For this review, take the finished solid that the model builds, in its own axes (mm). A direction names the side the tool comes from. Round coordinates to 2 decimals unless told otherwise and drop trailing zeros. Order: outer loops, then holes, each group sorted by start corner. A loop starts at its lowest first (then second) coordinate and runs counter-clockwise, first axis right, second up. Notation, with made-up numbers: (67.5, -36.5) -> (106.5, -36.5) arc R26 ccw to (106.5, 2.5) -> close; hole circle Ø10 at (35, 77.25). An arc over 180 degrees is marked (long way). Answer in a Markdown table with one row per item.
```python
from build123d import *

# Parameters (mm, degrees)
F1_DEPTH  = 93
F3_DEPTH  = 25
F4_W      = 122
F4_H      = 3
F4_W_2    = 15
F5_DEPTH  = 15
F6_DEPTH  = 15
F7_DEPTH  = 15
F8_DEPTH  = 15
F9_DEPTH  = 15
F10_DEPTH = 15
F11_DEPTH = 15
F12_DEPTH = 15
F13_DEPTH = 15
F14_DEPTH = 15
F15_DEPTH = 15
F16_DEPTH = 15
F17_DEPTH = 15
F18_DEPTH = 15
F19_W     = 10
F19_H     = 20
F20_DEPTH = 0.2
F21_R     = 2.5
F22_DEPTH = 2
F23_DEPTH = 2
F24_W     = 13
F24_H     = 5
F25_DEPTH = 2


with BuildPart() as f1:
    # F0 (on Top) → F1 (new body)
    with BuildSketch(Plane.XY):
        with BuildLine():
            Line((67.644592, 203.804426), (-232.355408, 203.804426))
            ThreePointArc((-232.355408, 203.804426), (-242.96201, 199.411027), (-247.355408, 188.804426))
            Line((-247.355408, 188.804426), (-247.355408, -176.195574))
            Line((-247.355408, -176.195574), (82.644592, -176.195574))
            Line((82.644592, -176.195574), (82.644592, 188.804426))
            ThreePointArc((82.644592, 188.804426), (78.251193, 199.411027), (67.644592, 203.804426))
        make_face()
        with BuildLine():
            ThreePointArc((-240.355408, 188.804426), (-238.012263, 194.46128), (-232.355408, 196.804426))
            Line((-232.355408, 196.804426), (67.644592, 196.804426))
            ThreePointArc((67.644592, 196.804426), (73.301446, 194.46128), (75.644592, 188.804426))
            Line((75.644592, 188.804426), (75.644592, -169.195574))
            Line((75.644592, -169.195574), (-240.355408, -169.195574))
            Line((-240.355408, -169.195574), (-240.355408, 188.804426))
        make_face(mode=Mode.SUBTRACT)
    extrude(amount=F1_DEPTH)

    # F2 (on face) → F3 (cut)
    with BuildSketch(Plane.XZ.offset(176.195574)):
        Polygon((-30.355408, 6), (72.644592, 6), (72.644592, 100.520082), (-30.355408, 100.520082), (-30.355408, 48), align=None)
        Polygon((-90.355408, 48), (-30.355408, 48), (-30.355408, 100.520082), (-90.355408, 99.808939), align=None)
    extrude(amount=-F3_DEPTH, mode=Mode.SUBTRACT)

    # F4 (on face) → F5 (cut)
    with BuildSketch(Plane(origin=(0, 203.804426, 0), x_dir=(-1, 0, 0), z_dir=(0, 1, 0))):
        with Locations((171.355408, 88.5)):
            Rectangle(F4_W, F4_H)
        with Locations((239.855408, 88.5)):
            Rectangle(F4_W_2, F4_H)
    extrude(amount=-F5_DEPTH, mode=Mode.SUBTRACT)

    # F4 (on face) → F6 (cut)
    with BuildSketch(Plane(origin=(0, 203.804426, 0), x_dir=(-1, 0, 0), z_dir=(0, 1, 0))):
        with Locations((171.355408, 82.5)):
            Rectangle(F4_W, F4_H)
        with Locations((239.855408, 82.5)):
            Rectangle(F4_W_2, F4_H)
    extrude(amount=-F6_DEPTH, mode=Mode.SUBTRACT)

    # F4 (on face) → F7 (cut)
    with BuildSketch(Plane(origin=(0, 203.804426, 0), x_dir=(-1, 0, 0), z_dir=(0, 1, 0))):
        with Locations((171.355408, 76.5)):
            Rectangle(F4_W, F4_H)
        with Locations((239.855408, 76.5)):
            Rectangle(F4_W_2, F4_H)
    extrude(amount=-F7_DEPTH, mode=Mode.SUBTRACT)

    # F4 (on face) → F8 (cut)
    with BuildSketch(Plane(origin=(0, 203.804426, 0), x_dir=(-1, 0, 0), z_dir=(0, 1, 0))):
        with Locations((171.355408, 70.5)):
            Rectangle(F4_W, F4_H)
        with Locations((239.855408, 70.5)):
            Rectangle(F4_W_2, F4_H)
    extrude(amount=-F8_DEPTH, mode=Mode.SUBTRACT)

    # F4 (on face) → F9 (cut)
    with BuildSketch(Plane(origin=(0, 203.804426, 0), x_dir=(-1, 0, 0), z_dir=(0, 1, 0))):
        with Locations((171.355408, 64.5)):
            Rectangle(F4_W, F4_H)
        with Locations((239.855408, 64.5)):
            Rectangle(F4_W_2, F4_H)
    extrude(amount=-F9_DEPTH, mode=Mode.SUBTRACT)

    # F4 (on face) → F10 (cut)
    with BuildSketch(Plane(origin=(0, 203.804426, 0), x_dir=(-1, 0, 0), z_dir=(0, 1, 0))):
        with Locations((171.355408, 58.5)):
            Rectangle(F4_W, F4_H)
        with Locations((239.855408, 58.5)):
            Rectangle(F4_W_2, F4_H)
    extrude(amount=-F10_DEPTH, mode=Mode.SUBTRACT)

    # F4 (on face) → F11 (cut)
    with BuildSketch(Plane(origin=(0, 203.804426, 0), x_dir=(-1, 0, 0), z_dir=(0, 1, 0))):
        with Locations((171.355408, 52.5)):
            Rectangle(F4_W, F4_H)
        with Locations((239.855408, 52.5)):
            Rectangle(F4_W_2, F4_H)
    extrude(amount=-F11_DEPTH, mode=Mode.SUBTRACT)

    # F4 (on face) → F12 (cut)
    with BuildSketch(Plane(origin=(0, 203.804426, 0), x_dir=(-1, 0, 0), z_dir=(0, 1, 0))):
        with Locations((171.355408, 46.5)):
            Rectangle(F4_W, F4_H)
        with Locations((239.855408, 46.5)):
            Rectangle(F4_W_2, F4_H)
    extrude(amount=-F12_DEPTH, mode=Mode.SUBTRACT)

    # F4 (on face) → F13 (cut)
    with BuildSketch(Plane(origin=(0, 203.804426, 0), x_dir=(-1, 0, 0), z_dir=(0, 1, 0))):
        with Locations((171.355408, 40.5)):
            Rectangle(F4_W, F4_H)
        with Locations((239.855408, 40.5)):
            Rectangle(F4_W_2, F4_H)
    extrude(amount=-F13_DEPTH, mode=Mode.SUBTRACT)

    # F4 (on face) → F14 (cut)
    with BuildSketch(Plane(origin=(0, 203.804426, 0), x_dir=(-1, 0, 0), z_dir=(0, 1, 0))):
        with Locations((171.355408, 34.5)):
            Rectangle(F4_W, F4_H)
        with Locations((239.855408, 34.5)):
            Rectangle(F4_W_2, F4_H)
    extrude(amount=-F14_DEPTH, mode=Mode.SUBTRACT)

    # F4 (on face) → F15 (cut)
    with BuildSketch(Plane(origin=(0, 203.804426, 0), x_dir=(-1, 0, 0), z_dir=(0, 1, 0))):
        with Locations((171.355408, 28.5)):
            Rectangle(F4_W, F4_H)
        with Locations((239.855408, 28.5)):
            Rectangle(F4_W_2, F4_H)
    extrude(amount=-F15_DEPTH, mode=Mode.SUBTRACT)

    # F4 (on face) → F16 (cut)
    with BuildSketch(Plane(origin=(0, 203.804426, 0), x_dir=(-1, 0, 0), z_dir=(0, 1, 0))):
        with Locations((171.355408, 22.5)):
            Rectangle(F4_W, F4_H)
        with Locations((239.855408, 22.5)):
            Rectangle(F4_W_2, F4_H)
    extrude(amount=-F16_DEPTH, mode=Mode.SUBTRACT)

    # F4 (on face) → F17 (cut)
    with BuildSketch(Plane(origin=(0, 203.804426, 0), x_dir=(-1, 0, 0), z_dir=(0, 1, 0))):
        with Locations((171.355408, 16.5)):
            Rectangle(F4_W, F4_H)
        with Locations((239.855408, 16.5)):
            Rectangle(F4_W_2, F4_H)
    extrude(amount=-F17_DEPTH, mode=Mode.SUBTRACT)

    # F4 (on face) → F18 (cut)
    with BuildSketch(Plane(origin=(0, 203.804426, 0), x_dir=(-1, 0, 0), z_dir=(0, 1, 0))):
        with Locations((171.355408, 10.5)):
            Rectangle(F4_W, F4_H)
        with Locations((239.855408, 10.5)):
            Rectangle(F4_W_2, F4_H)
    extrude(amount=-F18_DEPTH, mode=Mode.SUBTRACT)

    # F19 (on face) → F20 (join)
    with BuildSketch(Plane(origin=(0, 203.804426, 0), x_dir=(-1, 0, 0), z_dir=(0, 1, 0))):
        with Locations((88.355408, 73)):
            Rectangle(F19_W, F19_H)
    extrude(amount=F20_DEPTH)

    # F21 (on face) → F22 (cut)
    with BuildSketch(Plane(origin=(0, 203.804426, 0), x_dir=(-1, 0, 0), z_dir=(0, 1, 0))):
        with Locations((83.355408, 43)):
            Circle(F21_R)
    extrude(amount=-F22_DEPTH, mode=Mode.SUBTRACT)

    # F21 (on face) → F23 (cut)
    with BuildSketch(Plane(origin=(0, 203.804426, 0), x_dir=(-1, 0, 0), z_dir=(0, 1, 0))):
        with Locations((96.355408, 43)):
            Circle(F21_R)
    extrude(amount=-F23_DEPTH, mode=Mode.SUBTRACT)

    # F24 (on face) → F25 (cut)
    with BuildSketch(Plane(origin=(0, 203.804426, 0), x_dir=(-1, 0, 0), z_dir=(0, 1, 0))):
        with Locations((91.216292, 32.372116)):
            Rectangle(F24_W, F24_H)
    extrude(amount=-F25_DEPTH, mode=Mode.SUBTRACT)


solid = f1.part
```
Q1. The part is to be moulded in two halves that separate along X. For faces 1 (the face through (73.24, 194.52, 45.85)), 2 (the face through (-180, 200, 12)), 3 (the face through (-238.074, 194.399, 85.479)), 4 (the face through (-242.84, 199.53, 49.48)), say which applies: +X half, -X half, draft (parallel to the pull), parting line (faces both ways), or undercut.
Answer key:
| item | result |
|---|---|
| face 1 | undercut |
| face 2 | draft |
| face 3 | undercut |
| face 4 | -X half |
Q2. Clearance check with flat-ended pins moving along their axes: pin 1 Ø16.5 at (x, y) = (-199.5, 196.5) entering from -Z; pin 2 Ø10 at (x, z) = (-182, 54) entering from +Y; pin 3 Ø4.5 at (x, y) = (-180, 193) entering from +Z; pin 4 Ø3.5 at (y, z) = (201.5, 10.5) entering from -X. State where each tip first meets the part, or that it passes through.
Answer key:
| item | result |
|---|---|
| pin 1 | stops at z = 0 |
| pin 2 | stops at y = 203.8 |
| pin 3 | passes through |
| pin 4 | stops at x = -241.62 |
Q3. To check wall thickness, follow probe 1 along Y at (x, z) = (-126.5, 78.5); probe 2 along X at (y, z) = (105, 58.5); probe 3 along Y at (x, z) = (21, 8). State the ranges of each line that lie inside material, in increasing order.
Answer key:
| item | result |
|---|---|
| probe 1 | y = -176.2 to -169.2, 196.8 to 203.8 |
| probe 2 | x = -247.36 to -240.36, 75.64 to 82.64 |
| probe 3 | y = 196.8 to 203.8 |
Q4. Take a section at A-A, the plane x = 25.5. Write out the cut boundary in (y, z), then the cut area to 3 significant figures.
Answer key:
| item | result |
|---|---|
| outline | (-176.2, 0) -> (-169.2, 0) -> (-169.2, 6) -> (-176.2, 6) -> close; (196.8, 0) -> (203.8, 0) -> (203.8, 93) -> (196.8, 93) -> close |
| area | 693 mm^2 |
Q5. Take a section at C-C, the plane x = -226. Give the number of separate pieces and of enclosed holes in the cut face, then the cut area to 3 significant figures.
Answer key:
| item | result |
|---|---|
| separate pieces | 16 |
| enclosed holes | 0 |
| area | 1,010 mm^2 |
Q6. Take a section at B-B, the plane y = 178. Write out the cut boundary in (x, z), then the cut area to 3 significant figures.
Answer key:
| item | result |
|---|---|
| outline | (-247.36, 0) -> (-240.36, 0) -> (-240.36, 93) -> (-247.36, 93) -> close; (75.64, 0) -> (82.64, 0) -> (82.64, 93) -> (75.64, 93) -> close |
| area | 1,300 mm^2 |
Q7. Tool access review of faces 5 (the face through (-178, 200, 81)), 6 (the face through (-51, 196.804, 46)), 7 (the face through (-83, 198, 0)): name each direction out of +Z, -Z, +X, -X, +Y, -Y from which nothing blocks a thin tool from reaching the whole face with its end or side.
Answer key:
| item | result |
|---|---|
| face 5 | -X, +Y |
| face 6 | +Z, -Z |
| face 7 | -Z, +X, -X, +Y, -Y |
